```python
from build123d import *

# Parameters (mm, degrees)
SKETCH7_W           = 63.5
SKETCH7_H           = 3.175
BOSS_EXTRUDE4_DEPTH = 3.175
SKETCH8_R           = 2.2499955
CUT_EXTRUDE3_DEPTH  = 4.175
BOSS_EXTRUDE5_DEPTH = 6.35


with BuildPart() as part:
    # Sketch7 → Boss-Extrude4 (new body, symmetric)
    with BuildSketch(Plane(origin=(0, 0, 0), x_dir=(1, 0, 0), z_dir=(0, 1, 0))):
        Rectangle(SKETCH7_W, SKETCH7_H)
    extrude(amount=BOSS_EXTRUDE4_DEPTH, both=True)

    # Sketch8 → Cut-Extrude3 (cut, through all)
    with BuildSketch(Plane.XY.offset(1.5875)):
        with Locations((-25.4, 0)):
            Circle(SKETCH8_R)
        with Locations((25.4, 0)):
            Circle(SKETCH8_R)
    extrude(amount=-CUT_EXTRUDE3_DEPTH, mode=Mode.SUBTRACT)

    # Sketch9 → Boss-Extrude5 (add)
    with BuildSketch(Plane(origin=(0, 3.175, 0), x_dir=(1, 0, 0), z_dir=(0, 1, 0))):
        Polygon((19.05, -1.5875), (19.05, -33.3375), (-19.05, -1.5875), align=None)
    extrude(amount=-BOSS_EXTRUDE5_DEPTH)


solid = part.part
```
Model file for the job. Use its own axes, mm. A direction names the side the tool comes from. Coordinates: 2 decimals unless noted, no trailing zeros. Write each loop counter-clockwise with the first axis right and the second up, starting at its lowest first coordinate (ties: lowest second). Pieces come first, ordered by that corner, then holes. Notation, with made-up numbers: (34.25, -8.5) - (54.25, -8.5) arc R7 ccw to (54.25, -3.5) - close; hole circle Ø4 at (88, 59.25). An arc over 180 degrees is marked (long way). One line per question, with ' | ' between items. Start each with the question number.
Q1. Pull direction X, two halves, no side cores. Call faces 1 (the face through (31.75, 0, 0)), 2 (the face through (24, 2, 1.588)), 3 (the face through (27.546, 0.676, 0.022)): pulls with the +X half, pulls with the -X half, needs draft (parallel to the pull), parting line crosses it, or undercut.
Q2. Cut at C-C, the plane z = 10.5. List the corners of the cut face in (x, y) (3 decimals), then the cut area to 3 significant figures.
Q3. Pin check, flat tips, straight feed: pin 1 (1.5 mm diameter, centred on x = 6, y = 0, fed in from +Z); pin 2 (3 mm diameter, centred on y = 0, z = 28, fed in from -X) (3 decimals); pin 3 (1.5 mm diameter, centred on x = 22.5, y = -1.5, fed in from +Z). Stop position of each tip, or through.
Q4. Cut at B-B, the plane y = 0. List the corners of the cut face in (x, z), then the cut area to 3 significant figures.
Q5. Drill centre lines: line 1 (Y direction, x = -25.4, z = -0.25) (3 decimals); line 2 (Z direction, x = 23.5, y = 2.5); line 3 (X direction, y = 2.5, z = 21.5) (3 decimals). Where is each one in solid material? Low to high. Write a range as [from, to].
Q6. 3-axis set-ups, long thin cutter, end or side, ignore diameter. For faces 4 (the face through (19.05, 0, 17)), 5 (the face through (-27, 2, 1.588)), 6 (the face through (5, 3.175, 9)): which of +Z, -Z, +X, -X, +Y, -Y reach the whole face in a straight line?
Q7. Cut at D-D, the plane x = -18. List the corners of the cut face in (y, z) (1 decimal), then the cut area to 3 significant figures.
Answer below:
1) face 1: pulls with the +X half | face 2: needs draft | face 3: undercut
2) outline: (-8.355, -3.175) - (19.05, -3.175) - (19.05, 3.175) - (-8.355, 3.175) - close | area: 174 mm^2
3) pin 1: z = 23.09 | pin 2: x = 10.845 | pin 3: z = 1.59
4) outline: (-31.75, -1.59) - (-27.65, -1.59) - (-27.65, 1.59) - (-31.75, 1.59) - close; (-23.15, -1.59) - (23.15, -1.59) - (23.15, 1.59) - (19.05, 1.59) - (19.05, 33.34) - (-19.05, 1.59) - (-23.15, 1.59) - close; (27.65, -1.59) - (31.75, -1.59) - (31.75, 1.59) - (27.65, 1.59) - close | area: 778 mm^2
5) line 1: [-3.175, -2.25], [2.25, 3.175] | line 2: [-1.59, 1.59] | line 3: [4.845, 19.05]
6) face 4: +Z, +X, +Y, -Y | face 5: +Z, -X, +Y, -Y | face 6: +Z, -Z, +X, -X, +Y
7) outline: (-3.2, -1.6) - (3.2, -1.6) - (3.2, 2.5) - (-3.2, 2.5) - close | area: 25.7 mm^2
